from build123d import *

# Parameters (mm, degrees)
F1_DEPTH    = 13
F2_T1_DEPTH = 13
F3_R        = 0.2


# Not quite as in the source:
# - a fillet or chamfer that OpenCascade refuses, or shapes differently, is made with other operations: its cross-section is extruded or revolved along the edge and cut away or added
# - a feature names something its author has since deleted; it is built from what else it names


with BuildPart() as f1:
    # F0 (on Front) → F1 (new body)
    with BuildSketch(Plane.XZ):
        with BuildLine():
            Line((-3.4641016151, 1), (-17.5, 1))
            Line((-17.5, 1), (-17.5, -1))
            Line((-17.5, -1), (0, -1))
            ThreePointArc((0, -1), (-2, -0.4641016151), (-3.4641016151, 1))
        make_face()
        with BuildLine():
            ThreePointArc((-3.9382737335, 3.7), (-3.9397068673, 2.3081114255), (-3.4641016151, 1))
            Line((-3.4641016151, 1), (7e-09, 1))
            ThreePointArc((7e-09, 1), (-1.6431676705, 1.859824572), (-1.8734993995, 3.7))
            Line((-1.8734993995, 3.7), (-3.9382737335, 3.7))
        make_face()
        with BuildLine():
            Line((7e-09, 1), (-3.4641016151, 1))
            ThreePointArc((-3.4641016151, 1), (-2, -0.4641016151), (0, -1))
            ThreePointArc((0, -1), (2, -0.4641016151), (3.4641016151, 1))
            Line((3.4641016151, 1), (7e-09, 1))
        make_face()
        with BuildLine():
            ThreePointArc((1.8734993995, 3.7), (1.6431676745, 1.8598245778), (7e-09, 1))
            Line((7e-09, 1), (3.4641016151, 1))
            ThreePointArc((3.4641016151, 1), (3.9397068673, 2.3081114255), (3.9382737335, 3.7))
            Line((3.9382737335, 3.7), (1.8734993995, 3.7))
        make_face()
        with BuildLine():
            ThreePointArc((-3.8729833462, 4), (-3.9085079367, 3.8506266565), (-3.9382737335, 3.7))
            Line((-3.9382737335, 3.7), (-1.8734993995, 3.7))
            Line((-1.8734993995, 3.7), (-1.8734993995, 5))
            Line((-1.8734993995, 5), (-3.8729833462, 5))
            Line((-3.8729833462, 5), (-3.8729833462, 4))
        make_face()
        with BuildLine():
            ThreePointArc((3.4641016151, 1), (2, -0.4641016151), (0, -1))
            Line((0, -1), (17.5, -1))
            Line((17.5, -1), (17.5, 1))
            Line((17.5, 1), (3.4641016151, 1))
        make_face()
        with BuildLine():
            Line((1.8734993995, 5), (1.8734993995, 3.7))
            Line((1.8734993995, 3.7), (3.9382737335, 3.7))
            ThreePointArc((3.9382737335, 3.7), (3.9085079367, 3.8506266565), (3.8729833462, 4))
            Line((3.8729833462, 4), (3.8729833462, 5))
            Line((3.8729833462, 5), (1.8734993995, 5))
        make_face()
    extrude(amount=F1_DEPTH)

    # F2: fillet of radius 4 on 2 edges, made by hand

    # F2_s2 → F2_t1 (join)
    with BuildSketch(Plane.XZ):
        with BuildLine():
            ThreePointArc((-7.7459666924, 1), (-5.2964769496, 1.8377223398), (-3.8729833462, 4))
            ThreePointArc((-3.8729833462, 4), (-3.9633576589, 2.4598184865), (-3.4641016151, 1))
            Line((-3.4641016151, 1), (-7.7459666924, 1))
        make_face()
        with BuildLine():
            ThreePointArc((7.7459666924, 1), (5.2964769496, 1.8377223398), (3.8729833462, 4))
            ThreePointArc((3.8729833462, 4), (3.9633576589, 2.4598184865), (3.4641016151, 1))
            Line((3.4641016151, 1), (7.7459666924, 1))
        make_face()
    extrude(amount=F2_T1_DEPTH)

    # F3
    f3_edges = [f1.edges().sort_by_distance(p)[0] for p in [
        (-17.5, -6.5, 1),
        (17.5, -6.5, 1),
    ]]
    fillet(f3_edges, radius=F3_R)


solid = f1.part
Input: part model. Units: mm. Frame: model coordinates. A direction names the side the tool comes from. Coordinates: 2 decimals unless noted, no trailing zeros. Loops run counter-clockwise (first coordinate to the right, second up) from the corner with the lowest first, then second, coordinate; pieces in that order, holes last.
(1) Section B-B on z = 2.9. Return the cut outline in (x, y), then the cut area to 3 significant figures.
(2) Set-up query: faces 4 (the face through (1.873, -6, 4)), 5 (the face through (-12, -6, 1)), 6 (the face through (3.873, -6.4, 4.5)), 7 (the face through (3, -6, 5)). Return all of +Z, -Z, +X, -X, +Y, -Y with unobstructed straight access to the full face (end or side cutting, diameter ignored); none if empty.
(3) Section C-C on x = 13. Return the cut outline in (y, z).
(4) Pull-direction query (X, two-part tool) for faces 1 (the face through (0, -6, -1)), 2 (the face through (-1.873, -6, 4)), 3 (the face through (-3.873, -6.4, 4.5)); classes: released by +X, released by -X, zero draft, split by the parting line, or undercut.
(5) First-contact query: pin 1 Ø1.5 at (y, z) = (-7, 4) entering from +X; pin 2 Ø1 at (x, z) = (-0.5, 0.5) entering from +Y; pin 3 Ø5 at (x, y) = (14.5, -9.5) entering from +Z; pin 4 Ø1.5 at (y, z) = (-3.5, 3.5) entering from +X. Flat tips, straight axial feed; report the tip coordinate or a pass-through.
(6) Section A-A on y = -8.5. Return the cut outline in (x, z).
(7) Material intervals for probe 1 along X at (y, z) = (-11.5, 4.75); probe 2 along Z at (x, y) = (-9.5, -3.5); probe 3 along X at (y, z) = (-2.75, 1.9), sorted ascending.
(8) Section D-D on x = -7. Return the cut outline in (y, z).
Data:
1. outline: (-4.34, -13) - (-2, -13) - (-2, 0) - (-4.34, 0) - close; (2, -13) - (4.34, -13) - (4.34, 0) - (2, 0) - close
1. area: 60.9 mm2
2. face 4: +Z, +Y, -Y
2. face 5: +Z, -X, +Y, -Y
2. face 6: +Z, +X, +Y, -Y
2. face 7: +Z, +X, -X, +Y, -Y
3. outline: (-13, -1) - (0, -1) - (0, 1) - (-13, 1) - close
4. face 1: zero draft
4. face 2: undercut
4. face 3: released by -X
5. pin 1: stops at x = 4.15
5. pin 2: stops at y = 0
5. pin 3: stops at z = 1
5. pin 4: stops at x = 4.44
6. outline: (-17.5, -1) - (17.5, -1) - (17.5, 0.8) arc R0.2 ccw to (17.3, 1) - (7.75, 1) arc R4 cw to (3.87, 4) - (3.87, 5) - (1.87, 5) - (1.87, 3.7) arc R2 cw (long way) to (-1.87, 3.7) - (-1.87, 5) - (-3.87, 5) - (-3.87, 4) arc R4 cw to (-7.75, 1) - (-17.3, 1) arc R0.2 ccw to (-17.5, 0.8) - close
7. probe 1: x = -3.87 to -1.87, 1.87 to 3.87
7. probe 2: z = -1 to 1
7. probe 3: x = -5.22 to -1.67, 1.67 to 5.22
8. outline: (-13, -1) - (0, -1) - (0, 1.07) - (-13, 1.07) - close
